Source: CAD feature listing. Evaluate the final solid. Frame: model axes, mm. A direction names the side the tool comes from. Coordinates: 2 decimals unless noted, no trailing zeros. Write each loop counter-clockwise with the first axis right and the second up, starting at its lowest first coordinate (ties: lowest second). Pieces come first, ordered by that corner, then holes. Notation, with made-up numbers: M 55,0.25 L 85,0.25 A4 cw 85,6.25 Z; hole C -18.75,-37 d5. An arc over 180 degrees is marked long. Write item = value, one per line. Start each with the question number.
1. Pull-direction query (Z, two-part tool) for faces 4 (the face through (67.464, 0.246, 112.989)), 5 (the face through (-2.66, 0.25, 116.88)), 6 (the face through (33, 4, 4.125)), 7 (the face through (68.638, 0.263, 110.595)); classes: pulls with the +Z half, pulls with the -Z half, needs draft (parallel to the pull), parting line crosses it, or undercut.
2. Section query B-B (z = 13.5). Output: boundary loops of the cut face in (x, y).
3. Line query: line 1 along X through (y, z) = (0.3, 0); line 2 along Z through (x, y) = (66, 0.45) (3 decimals); line 3 along Z through (x, y) = (12, 4.5) (3 decimals). Output: solid intervals per line, ascending.
4. Access query for faces 1 (the face through (33, 4, 109.625)), 2 (the face through (-2.638, 0.263, 110.595)), 3 (the face through (68.638, 0.263, 3.155)). Directions: +Z, -Z, +X, -X, +Y, -Y. A direction counts if a zero-diameter tool reaches every point of the face in a straight line with its end or side. Return the directions, or none.
5. Section query C-C (y = 2.75). Output: boundary loops of the cut face in (x, z) (3 decimals).
6. Pin query (flat end, axial travel): pin 1 Ø3.5 at (y, z) = (4.5, 56) entering from -X; pin 2 Ø10 at (x, z) = (42.5, 20.5) entering from -Y; pin 3 Ø4 at (x, z) = (47.5, -1.5) entering from +Y; pin 4 Ø5 at (x, y) = (4, 7) entering from +Z (3 decimals). Return the tip coordinate at first contact, or that it passes through.
7. Section query A-A (x = 17). Output: boundary loops of the cut face in (y, z) (3 decimals), then the cut area to 3 significant figures.
```python
from build123d import *

# Parameters (mm, degrees)
SKETCH_1_R      = 1.65
EXTRUDE_1_DEPTH = 0.5
FILLET_1_R      = 3.3
SKETCH_2_W      = 66.770552446
SKETCH_2_H      = 105.5
EXTRUDE_2_DEPTH = 6.83
FILLET_2_R      = 1
EXTRUDE_3_DEPTH = 1.78
FILLET_3_R      = 1


with BuildPart() as part:
    # 草图1 → 凸台-拉伸1 (new body)
    with BuildSketch(Plane(origin=(0, 0, 0), x_dir=(1, 0, 0), z_dir=(0, 1, 0))):
        Polygon((66.385276223, -4.125), (69.6, -4.125), (69.6, 4.125), (-3.6, 4.125), (-3.6, -4.125), (-0.385276223, -4.125), (-0.385276223, -109.625), (-3.6, -109.625), (-3.6, -117.875), (69.6, -117.875), (69.6, -109.625), (66.385276223, -109.625), align=None)
        with Locations(Location((0, 0, 0), (0, 0, 270))):
            Circle(SKETCH_1_R, mode=Mode.SUBTRACT)
        with Locations(Location((66, 0, 0), (0, 0, 270))):
            Circle(SKETCH_1_R, mode=Mode.SUBTRACT)
        with Locations(Location((66, -113.75, 0), (0, 0, 90))):
            Circle(SKETCH_1_R, mode=Mode.SUBTRACT)
        with Locations(Location((0, -113.75, 0), (0, 0, 90))):
            Circle(SKETCH_1_R, mode=Mode.SUBTRACT)
    extrude(amount=EXTRUDE_1_DEPTH)

    # 圆角1
    # the kernel refuses this fillet: 3.3 mm, written as the material it takes off along each edge
    with BuildSketch(Plane(origin=(69.6, -8.247244982, 109.625), x_dir=(0, 0, 1), z_dir=(0, 1, 0)), Plane(origin=(-3.6, -8.247244982, 4.125), x_dir=(0, 0, -1), z_dir=(0, 1, 0))) as fillet_1_piece_1:
        with BuildLine():
            CenterArc((3.298897993, -3.3), FILLET_1_R, 90, 88.519238897)
            Line((0, -3.214723777), (-0.06597796, -3.213018252))
            ThreePointArc((-0.06597796, -3.213018252), (-0.066, -1.607361888), (-0.066, 0))
            Line((-0.066, 0), (0, 0.066))
            Line((0, 0.066), (3.298897993, 0.066))
            Line((3.298897993, 0.066), (3.298897993, 0))
        make_face()
    extrude(amount=16.994489963, mode=Mode.SUBTRACT)
    with BuildSketch(Plane(origin=(69.6, -8.25, 117.875), x_dir=(-1, 0, 0), z_dir=(0, 1, 0)), Plane(origin=(-3.6, -8.25, 117.875), x_dir=(0, 0, -1), z_dir=(0, 1, 0)), Plane(origin=(-3.6, -8.25, -4.125), x_dir=(1, 0, 0), z_dir=(0, 1, 0)), Plane(origin=(69.6, -8.25, -4.125), x_dir=(0, 0, 1), z_dir=(0, 1, 0))) as fillet_1_piece_2:
        with BuildLine():
            CenterArc((FILLET_1_R, -FILLET_1_R), FILLET_1_R, 90, 90)
            Line((0, -FILLET_1_R), (-FILLET_1_R * 0.02, -FILLET_1_R))
            Line((-FILLET_1_R * 0.02, -FILLET_1_R), (-FILLET_1_R * 0.02, FILLET_1_R * 0.02))
            Line((-FILLET_1_R * 0.02, FILLET_1_R * 0.02), (FILLET_1_R, FILLET_1_R * 0.02))
            Line((FILLET_1_R, FILLET_1_R * 0.02), (FILLET_1_R, 0))
        make_face()
    extrude(amount=17, mode=Mode.SUBTRACT)
    with BuildSketch(Plane(origin=(-3.6, -8.247244982, 109.625), x_dir=(1, 0, 0), z_dir=(0, 1, 0)), Plane(origin=(69.6, -8.247244982, 4.125), x_dir=(-1, 0, 0), z_dir=(0, 1, 0))) as fillet_1_piece_3:
        with BuildLine():
            CenterArc((3.3, -3.298897993), FILLET_1_R, 91.480761103, 88.519238897)
            Line((0, -3.298897993), (-0.066, -3.298897993))
            Line((-0.066, -3.298897993), (-0.066, 0))
            Line((-0.066, 0), (0, 0.066))
            ThreePointArc((0, 0.066), (1.607361888, 0.066), (3.213018252, 0.06597796))
            Line((3.213018252, 0.06597796), (3.214723777, 0))
        make_face()
    extrude(amount=16.994489963, mode=Mode.SUBTRACT)

    # 草图2 → 凸台-拉伸2 (add)
    with BuildSketch(Plane(origin=(0, 0, 0), x_dir=(1, 0, 0), z_dir=(0, 1, 0))):
        with Locations((33, -56.875)):
            Rectangle(SKETCH_2_W, SKETCH_2_H)
    extrude(amount=EXTRUDE_2_DEPTH)

    # 圆角2
    fillet_2_edges = [part.edges().sort_by_distance(p)[0] for p in [
        (-0.385276223, 3.665, 4.125),
        (-0.385276223, 3.665, 109.625),
        (66.385276223, 3.665, 109.625),
        (66.385276223, 3.665, 4.125),
    ]]
    fillet(fillet_2_edges, radius=FILLET_2_R)

    # 草图3 → 凸台-拉伸3 (add)
    with BuildSketch(Plane(origin=(0, 6.83, 0), x_dir=(1, 0, 0), z_dir=(0, 1, 0))):
        with BuildLine():
            Line((66.185276223, -108.625), (66.185276223, -5.125))
            ThreePointArc((66.185276223, -5.125), (65.950961648, -4.559314575), (65.385276223, -4.325))
            Line((65.385276223, -4.325), (0.614723777, -4.325))
            ThreePointArc((0.614723777, -4.325), (0.049038352, -4.559314575), (-0.185276223, -5.125))
            Line((-0.185276223, -5.125), (-0.185276223, -108.625))
            ThreePointArc((-0.185276223, -108.625), (0.049038352, -109.190685425), (0.614723777, -109.425))
            Line((0.614723777, -109.425), (65.385276223, -109.425))
            ThreePointArc((65.385276223, -109.425), (65.950961648, -109.190685425), (66.185276223, -108.625))
        make_face()
    extrude(amount=EXTRUDE_3_DEPTH)

    # 圆角3
    # the kernel refuses this fillet: 1 mm, written as the material it adds along each edge
    with BuildSketch(Plane(origin=(65.385276223, 0.5, 108.625), x_dir=(-0.8017442392976621, 0, -0.5976672776328089), z_dir=(-0.5976672776328089, 0, 0.8017442392976621))) as fillet_3_piece_1_section:
        with BuildLine():
            CenterArc((1 + FILLET_3_R, -FILLET_3_R), FILLET_3_R, 90, 90)
            Line((1 + FILLET_3_R, 0), (1, 0))
            Line((1, 0), (1, -FILLET_3_R))
        make_face()
    fillet_3_piece_1 = revolve(axis=Axis((65.385276223, 0.5, 108.625), (0, -1, 0)), revolution_arc=233.296989237, mode=Mode.PRIVATE)
    fillet_3_piece_1 = split(fillet_3_piece_1, bisect_by=Plane(origin=(66.385276223, 0.811675846, 109.374877518), z_dir=(-1, 0, 0)), keep=Keep.TOP, mode=Mode.PRIVATE)
    add(fillet_3_piece_1)
    with BuildSketch(Plane(origin=(65.385276223, 0.5, 108.625), x_dir=(-0.8017442392976621, 0, -0.5976672776328089), z_dir=(-0.5976672776328089, 0, 0.8017442392976621))) as fillet_3_piece_2_section:
        with BuildLine():
            CenterArc((1 + FILLET_3_R, -FILLET_3_R), FILLET_3_R, 90, 90)
            Line((1 + FILLET_3_R, 0), (1, 0))
            Line((1, 0), (1, -FILLET_3_R))
        make_face()
    fillet_3_piece_2 = revolve(axis=Axis((65.385276223, 0.5, 108.625), (0, -1, 0)), revolution_arc=233.296989237, mode=Mode.PRIVATE)
    fillet_3_piece_2 = fillet_3_piece_2 & Plane(origin=(66.3, 0.537437966, 112.923897993), x_dir=(0, 0, 1), z_dir=(0, -1, 0)) * Cylinder(3.3, 8, mode=Mode.PRIVATE)
    add(fillet_3_piece_2)
    with BuildSketch(Plane(origin=(0.614723777, 0.5, 108.625), x_dir=(0.8017442392976509, 0, -0.597667277632824), z_dir=(0.597667277632824, 0, 0.8017442392976509))) as fillet_3_piece_3_section:
        with BuildLine():
            CenterArc((1 + FILLET_3_R, FILLET_3_R), FILLET_3_R, 180, 90)
            Line((1, FILLET_3_R), (1, 0))
            Line((1, 0), (1 + FILLET_3_R, 0))
        make_face()
    fillet_3_piece_3 = revolve(axis=Axis((0.614723777, 0.5, 108.625), (0, 1, 0)), revolution_arc=233.296989237, mode=Mode.PRIVATE)
    fillet_3_piece_3 = split(fillet_3_piece_3, bisect_by=Plane(origin=(-0.385276223, 0.811675592, 109.374877608), z_dir=(1, 0, 0)), keep=Keep.TOP, mode=Mode.PRIVATE)
    add(fillet_3_piece_3)
    with BuildSketch(Plane(origin=(0.614723777, 0.5, 108.625), x_dir=(0.8017442392976509, 0, -0.597667277632824), z_dir=(0.597667277632824, 0, 0.8017442392976509))) as fillet_3_piece_4_section:
        with BuildLine():
            CenterArc((1 + FILLET_3_R, FILLET_3_R), FILLET_3_R, 180, 90)
            Line((1, FILLET_3_R), (1, 0))
            Line((1, 0), (1 + FILLET_3_R, 0))
        make_face()
    fillet_3_piece_4 = revolve(axis=Axis((0.614723777, 0.5, 108.625), (0, 1, 0)), revolution_arc=233.296989237, mode=Mode.PRIVATE)
    fillet_3_piece_4 = fillet_3_piece_4 & Plane(origin=(-0.3, 0.537437971, 112.923897993), x_dir=(1, 0, 0), z_dir=(0, -1, 0)) * Cylinder(3.3, 8, mode=Mode.PRIVATE)
    add(fillet_3_piece_4)
    with BuildSketch(Plane(origin=(0.614723777, 0.5, 5.125), x_dir=(0.8017442392976485, 0, 0.5976672776328273), z_dir=(0.5976672776328273, 0, -0.8017442392976485))) as fillet_3_piece_5_section:
        with BuildLine():
            CenterArc((1 + FILLET_3_R, -FILLET_3_R), FILLET_3_R, 90, 90)
            Line((1, -FILLET_3_R), (1, 0))
            Line((1, 0), (1 + FILLET_3_R, 0))
        make_face()
    fillet_3_piece_5 = revolve(axis=Axis((0.614723777, 0.5, 5.125), (0, -1, 0)), revolution_arc=233.296989237, mode=Mode.PRIVATE)
    fillet_3_piece_5 = split(fillet_3_piece_5, bisect_by=Plane(origin=(-0.385276223, 0.811675846, 4.375122482), z_dir=(1, 0, 0)), keep=Keep.TOP, mode=Mode.PRIVATE)
    add(fillet_3_piece_5)
    with BuildSketch(Plane(origin=(0.614723777, 0.5, 5.125), x_dir=(0.8017442392976485, 0, 0.5976672776328273), z_dir=(0.5976672776328273, 0, -0.8017442392976485))) as fillet_3_piece_6_section:
        with BuildLine():
            CenterArc((1 + FILLET_3_R, -FILLET_3_R), FILLET_3_R, 90, 90)
            Line((1, -FILLET_3_R), (1, 0))
            Line((1, 0), (1 + FILLET_3_R, 0))
        make_face()
    fillet_3_piece_6 = revolve(axis=Axis((0.614723777, 0.5, 5.125), (0, -1, 0)), revolution_arc=233.296989237, mode=Mode.PRIVATE)
    fillet_3_piece_6 = fillet_3_piece_6 & Plane(origin=(-0.3, 0.537437966, 0.826102007), x_dir=(0, 0, -1), z_dir=(0, -1, 0)) * Cylinder(3.3, 8, mode=Mode.PRIVATE)
    add(fillet_3_piece_6)
    with BuildSketch(Plane(origin=(65.385276223, 0.5, 5.125), x_dir=(-0.801744239297651, 0, 0.5976672776328237), z_dir=(-0.5976672776328237, 0, -0.801744239297651))) as fillet_3_piece_7_section:
        with BuildLine():
            CenterArc((1 + FILLET_3_R, FILLET_3_R), FILLET_3_R, 180, 90)
            Line((1 + FILLET_3_R, 0), (1, 0))
            Line((1, 0), (1, FILLET_3_R))
        make_face()
    fillet_3_piece_7 = revolve(axis=Axis((65.385276223, 0.5, 5.125), (0, 1, 0)), revolution_arc=233.296989237, mode=Mode.PRIVATE)
    fillet_3_piece_7 = split(fillet_3_piece_7, bisect_by=Plane(origin=(66.385276223, 0.811675555, 4.375122379), z_dir=(-1, 0, 0)), keep=Keep.TOP, mode=Mode.PRIVATE)
    add(fillet_3_piece_7)
    with BuildSketch(Plane(origin=(65.385276223, 0.5, 5.125), x_dir=(-0.801744239297651, 0, 0.5976672776328237), z_dir=(-0.5976672776328237, 0, -0.801744239297651))) as fillet_3_piece_8_section:
        with BuildLine():
            CenterArc((1 + FILLET_3_R, FILLET_3_R), FILLET_3_R, 180, 90)
            Line((1 + FILLET_3_R, 0), (1, 0))
            Line((1, 0), (1, FILLET_3_R))
        make_face()
    fillet_3_piece_8 = revolve(axis=Axis((65.385276223, 0.5, 5.125), (0, 1, 0)), revolution_arc=233.296989237, mode=Mode.PRIVATE)
    fillet_3_piece_8 = fillet_3_piece_8 & Plane(origin=(66.3, 0.537437971, 0.826102007), x_dir=(-1, 0, 0), z_dir=(0, -1, 0)) * Cylinder(3.3, 8, mode=Mode.PRIVATE)
    add(fillet_3_piece_8)
    with BuildSketch(Plane(origin=(0.614723777, 0.5, 109.625), x_dir=(0, 0, 1), z_dir=(1, 0, 0)), Plane(origin=(65.385276223, 0.5, 4.125), x_dir=(0, 0, -1), z_dir=(-1, 0, 0))) as fillet_3_piece_9:
        with BuildLine():
            CenterArc((FILLET_3_R, -FILLET_3_R), FILLET_3_R, 90, 90)
            Line((0, -FILLET_3_R), (0, 0))
            Line((0, 0), (FILLET_3_R, 0))
        make_face()
    extrude(amount=64.770552447)


solid = part.part
```
Results are:
q1.face_4 = undercut
q1.face_5 = pulls with the +Z half
q1.face_6 = pulls with the -Z half
q1.face_7 = undercut
q2.outline = M -0.39,0 L 66.39,0 L 66.39,6.83 L 66.19,6.83 L 66.19,8.61 L -0.19,8.61 L -0.19,6.83 L -0.39,6.83 Z
q3.line_1 = -3.6 to -1.65, 1.65 to 64.35, 67.65 to 69.6
q3.line_2 = -4.125 to -1.65, 1.65 to 112.1, 115.4 to 117.875
q3.line_3 = 4.125 to 109.625
q4.face_1 = +Z, +X, -X, +Y
q4.face_2 = -X, +Y, -Y
q4.face_3 = +X, +Y, -Y
q5.outline = M -0.385,5.125 A1 ccw 0.615,4.125 L 65.385,4.125 A1 ccw 66.385,5.125 L 66.385,108.625 A1 ccw 65.385,109.625 L 0.615,109.625 A1 ccw -0.385,108.625 Z
q6.pin_1 = -0.39
q6.pin_2 = 0
q6.pin_3 = 0.5
q6.pin_4 = 109.625
q7.outline = M 0,-4.125 L 0.5,-4.125 L 0.5,3.125 A1 cw 1.5,4.125 L 6.83,4.125 L 6.83,4.325 L 8.61,4.325 L 8.61,109.425 L 6.83,109.425 L 6.83,109.625 L 1.5,109.625 A1 cw 0.5,110.625 L 0.5,117.875 L 0,117.875 Z
q7.area = 916 mm^2
